Geometry check sheet. Reference: the model listing, model coordinates, mm. Face numbers are marked on the shaded views. A direction names the side the tool comes from. Give positions to 0.01 mm unless a question says otherwise; leave off trailing zeros. Order: outer loops, then holes, each group sorted by start corner. A loop starts at its lowest first (then second) coordinate and runs counter-clockwise, first axis right, second up. Notation, with made-up numbers: M -38.5,82.25 L -32.5,82.25 A20 ccw -32.5,113.25 Z; hole C 80.25,-29 d9. An arc over 180 degrees is marked long. Answer as CSV lines item,"result". Start each with the question number.
Q1. Thickness scan on line 1 (Y direction, x = 38, z = 16); line 2 (X direction, y = -38.1, z = 46.75); line 3 (X direction, y = -37.5, z = 24). Record the ranges inside material, lowest first.
Q2. Go/stop test with flat-tipped pins: pin 1 (14.5 mm diameter, centred on y = -38.1, z = 38.1, fed in from +X); pin 2 (5 mm diameter, centred on y = -56, z = 24, fed in from -X); pin 3 (1.5 mm diameter, centred on x = 105, y = -68, fed in from +Z). Record where each tip stops, or that it passes through.
Q3. Set-up check for the marked faces 1 and 2: record each of +Z, -Z, +X, -X, +Y, -Y from which the full face is reachable in a straight line by a thin tool's end or side.
Q4. Section check B-B, the plane z = 30. Record the boundary of the cut face in (x, y), then the cut area to 3 significant figures.
Q5. Section check A-A, the plane y = -38.1. Record the boundary of the cut face in (x, z).
Q6. Mould release check, pull along Y, two halves, no side actions. Record for the marked faces 3, 4 and 5: +Y half, -Y half, draft (parallel to the pull), parting line (faces both ways), or undercut.
Q7. Section check C-C, the plane x = 8.5. Record the boundary of the cut face in (y, z).
Q8. Section check D-D, the plane y = -64.5. Record the boundary of the cut face in (x, z).
```python
from build123d import *

# Parameters (mm, degrees)
F1_DEPTH = 76.2
F4_D     = 12.7
F5_D     = 12.7


with BuildPart() as f1:
    # F0 (on Front) → F1 (new body)
    with BuildSketch(Plane.XZ):
        Polygon((0, 50.8), (0, 0), (127, 0), (127, 25.4), (76.2, 25.4), (76.2, 50.8), (55.7977, 50.8), align=None)
    extrude(amount=F1_DEPTH)

    # F4 (through all)
    with Locations(Plane.XY.offset(50.8)):
        with Locations((38.1, -38.1)):
            Hole(F4_D / 2)

    # F5 (through all)
    with Locations(Plane.YZ.offset(76.2)):
        with Locations((-38.1, 38.1)):
            Hole(F5_D / 2)


solid = f1.part
```
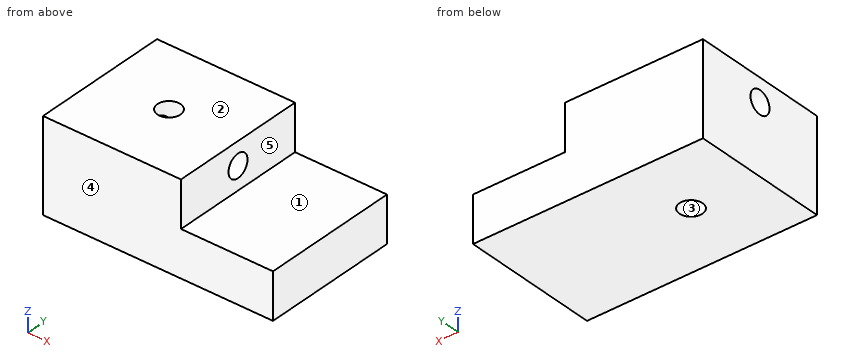
Answer block:
1,line 1,"y = -76.2 to -44.45, -31.75 to 0"
1,line 2,"x = 0 to 31.75, 44.45 to 76.2"
1,line 3,"x = 0 to 31.78, 44.42 to 127"
2,pin 1,"stops at x = 76.2"
2,pin 2,"stops at x = 0"
2,pin 3,"stops at z = 25.4"
3,face 1,"+Z, +X, +Y, -Y"
3,face 2,"+Z, +X, -X, +Y, -Y"
4,outline,"M 0,-76.2 L 76.2,-76.2 L 76.2,0 L 0,0 Z; hole C 38.1,-38.1 d12.7"
4,area,"5,680 mm2"
5,outline,"M 0,0 L 31.75,0 L 31.75,31.75 L 0,31.75 Z; M 0,44.45 L 31.75,44.45 L 31.75,50.8 L 0,50.8 Z; M 44.45,0 L 127,0 L 127,25.4 L 76.2,25.4 L 76.2,31.75 L 44.45,31.75 Z; M 44.45,44.45 L 76.2,44.45 L 76.2,50.8 L 44.45,50.8 Z"
6,face 3,"undercut"
6,face 4,"-Y half"
6,face 5,"draft"
7,outline,"M -76.2,0 L 0,0 L 0,50.8 L -76.2,50.8 Z; hole C -38.1,38.1 d12.7"
8,outline,"M 0,0 L 127,0 L 127,25.4 L 76.2,25.4 L 76.2,50.8 L 0,50.8 Z"
